from build123d import *

# Parameters (mm, degrees)
BOSS_EXTRUDE1_DEPTH   = 3.81
F_4_40_TAPPED_HOLE1_D = 2.2606
CUT_EXTRUDE1_DEPTH    = 4.81
SKETCH5_R             = 1.5875
CUT_EXTRUDE2_DEPTH    = 4.81
FILLET1_R             = 3


with BuildPart() as part:
    # Sketch1 → Boss-Extrude1 (new body)
    with BuildSketch(Plane(origin=(0, 0, 0), x_dir=(1, 0, 0), z_dir=(0, 1, 0))):
        with BuildLine():
            Line((0.307655172, 6.517241379), (0.307655172, -26.502758621))
            ThreePointArc((0.307655172, -26.502758621), (4.498655172, -30.693758621), (8.689655172, -26.502758621))
            Line((8.689655172, -26.502758621), (8.689655172, 6.517241379))
            ThreePointArc((8.689655172, 6.517241379), (4.498655172, 10.708241379), (0.307655172, 6.517241379))
        make_face()
    extrude(amount=BOSS_EXTRUDE1_DEPTH)

    # #4-40 Tapped Hole1 (through all)
    with Locations(Plane(origin=(0, 3.81, 0), x_dir=(1, 0, 0), z_dir=(0, 1, 0))):
        with Locations((4.498655172, 6.517241379), (4.498655172, -26.502758621)):
            Hole(F_4_40_TAPPED_HOLE1_D / 2)

    # Sketch4 → Cut-Extrude1 (cut, through all)
    with BuildSketch(Plane(origin=(0, 3.81, 0), x_dir=(1, 0, 0), z_dir=(0, 1, 0))):
        with BuildLine():
            Line((-105.054689706, 41.50252919), (-22.868233876, -25.472974727))
            ThreePointArc((-22.868233876, -25.472974727), (0.331829627, -23.107123199), (-2.0340219, 0.092940304))
            Line((-2.0340219, 0.092940304), (-84.220477731, 67.068444221))
            Line((-84.220477731, 67.068444221), (-248.593389391, 201.019452054))
            Line((-248.593389391, 201.019452054), (-269.427601367, 175.453537024))
            Line((-269.427601367, 175.453537024), (-105.054689706, 41.50252919))
        make_face()
    extrude(amount=-CUT_EXTRUDE1_DEPTH, mode=Mode.SUBTRACT)

    # Sketch5 → Cut-Extrude2 (cut, through all)
    with BuildSketch(Plane(origin=(0, 3.81, 0), x_dir=(1, 0, 0), z_dir=(0, 1, 0))):
        with Locations((4.498655172, 6.517241379)):
            Circle(SKETCH5_R)
    extrude(amount=-CUT_EXTRUDE2_DEPTH, mode=Mode.SUBTRACT)

    # Fillet1
    fillet1_edges = [part.edges().sort_by_distance(p)[0] for p in [
        (0.307655172, 1.905, 23.136717878),
        (0.307655172, 1.905, 2.243316545),
    ]]
    fillet(fillet1_edges, radius=FILLET1_R)


solid = part.part
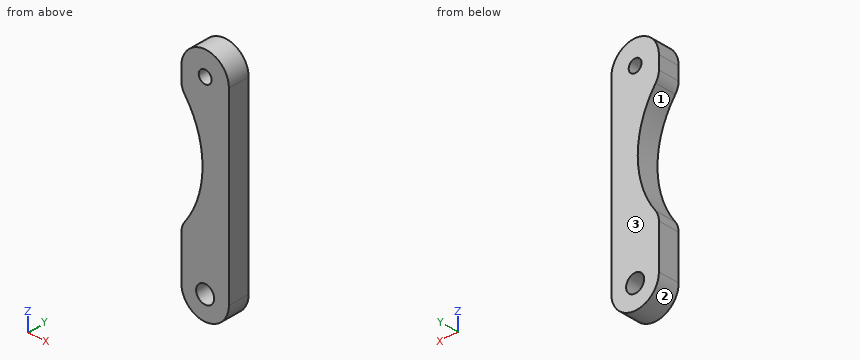
Can you work these out from the model? Positions are in its coordinate system, mm. Face numbers are marked on the shaded views. Round coordinates to 2 decimals unless told otherwise and drop trailing zeros. Write each loop counter-clockwise with the first axis right and the second up, starting at its lowest first coordinate (ties: lowest second). Pieces come first, ordered by that corner, then holes. Notation, with made-up numbers: M 73.5,72.25 L 102.5,72.25 A11 cw 102.5,87.25 Z; hole C 54,34.25 d10. An arc over 180 degrees is marked long. Use a Markdown table: item, result.
Item 1: I want a section at A-A (y = 1). List the corners of the cut face in (x, z) for me (1 decimal).
Found:
| item | result |
|---|---|
| outline | M 0.3,-6.5 A4.2 ccw 8.7,-6.5 L 8.7,26.5 A4.2 ccw 0.3,26.5 L 0.3,24.2 A3 ccw 0.9,22.4 A16.5 cw 0.9,3 A3 ccw 0.3,1.2 Z; hole C 4.5,-6.5 d3.2; hole C 4.5,26.5 d2.3 |
Item 2: If I drill on line 1 along Z through (x, y) = (4.5, 2.35); line 2 along Z through (x, y) = (5.25, 0.9); line 3 along X through (y, z) = (3.3, 12.5), over which ranges is the centre line in solid material (lowest first)? Write a range as [from, to].
Found:
| item | result |
|---|---|
| line 1 | z = [-10.71, -8.1], [-4.93, 25.37], [27.63, 30.69] |
| line 2 | z = [-10.64, -7.92], [-5.12, 25.66], [27.35, 30.63] |
| line 3 | x = [4.04, 8.69] |
Item 3: For pin 1 Ø1.9 at (x, z) = (4.5, -6.52) entering from -Y, with a flat end and sliding along its axis, tell me the tip position at first contact or that it passes through.
Found:
| item | result |
|---|---|
| pin 1 | passes through |
Item 4: I want a section at C-C (z = -7). List the corners of the cut face in (x, y) for me, and give its area (3 significant figures).
Found:
| item | result |
|---|---|
| outline | M 0.34,0 L 2.99,0 L 2.99,3.81 L 0.34,3.81 Z; M 6.01,0 L 8.66,0 L 8.66,3.81 L 6.01,3.81 Z |
| area | 20.2 mm2 |
Item 5: I want a section at D-D (x = 8). List the corners of the cut face in (y, z) for me.
Found:
| item | result |
|---|---|
| outline | M 0,-8.82 L 3.81,-8.82 L 3.81,28.81 L 0,28.81 Z |
Item 6: We'd pull the mould along Z, two halves only. Please class the marked faces 1, 2 and 3: released by +Z, released by -Z, zero draft, split by the parting line, or undercut.
Found:
| item | result |
|---|---|
| face 1 | undercut |
| face 2 | released by -Z |
| face 3 | zero draft |
Item 7: I want a section at B-B (x = 1.5). List the corners of the cut face in (y, z) for me, and give its area (3 significant figures).
Found:
| item | result |
|---|---|
| outline | M 0,-9.45 L 3.81,-9.45 L 3.81,3.9 L 0,3.9 Z; M 0,21.48 L 3.81,21.48 L 3.81,29.43 L 0,29.43 Z |
| area | 81.1 mm2 |
